```python
from build123d import *

# Parameters (mm, degrees)
SKETCH1_W           = 76.2
SKETCH1_H           = 25.4
SKETCH1_W_2         = 69.85
SKETCH1_H_2         = 19.05
EXTRUDE_THIN1_DEPTH = 38.1
SKETCH2_R           = 3.175
CUT_EXTRUDE1_DEPTH  = 77.2
SKETCH3_R           = 24.97201
CUT_EXTRUDE2_DEPTH  = 26.4


with BuildPart() as part:
    # Sketch1 → Extrude-Thin1 (new body, symmetric)
    with BuildSketch(Plane.XY):
        Rectangle(SKETCH1_W, SKETCH1_H)
        Rectangle(SKETCH1_W_2, SKETCH1_H_2, mode=Mode.SUBTRACT)
    extrude(amount=EXTRUDE_THIN1_DEPTH, both=True)

    # Sketch2 → Cut-Extrude1 (cut, through all)
    with BuildSketch(Plane.ZY.offset(38.1)):
        Circle(SKETCH2_R)
    extrude(amount=-CUT_EXTRUDE1_DEPTH, mode=Mode.SUBTRACT)

    # Sketch3 → Cut-Extrude2 (cut, through all)
    with BuildSketch(Plane(origin=(0, 12.7, 0), x_dir=(1, 0, 0), z_dir=(0, 1, 0))):
        Circle(SKETCH3_R)
    extrude(amount=-CUT_EXTRUDE2_DEPTH, mode=Mode.SUBTRACT)


solid = part.part
```
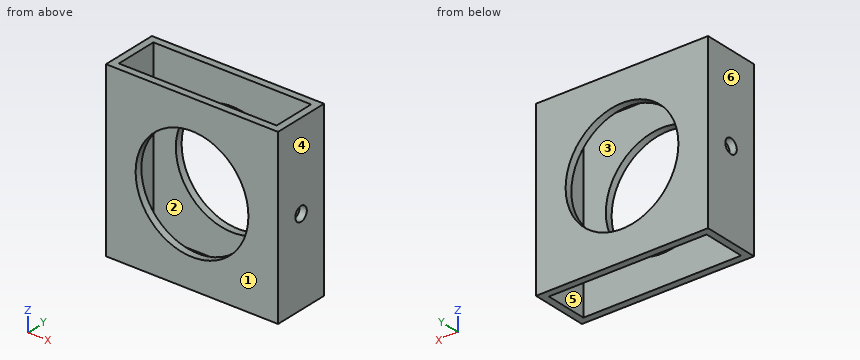
Design review of the part built by this model. Coordinates are the model's own, in mm. Face numbers are marked on the shaded views. A direction names the side the tool comes from. Coordinates: 2 decimals unless noted, no trailing zeros. Order: outer loops, then holes, each group sorted by start corner. A loop starts at its lowest first (then second) coordinate and runs counter-clockwise, first axis right, second up. Notation, with made-up numbers: (-8, 50.25) -> (32, 50.25) arc R27 cw to (32, 85.25) -> close; hole circle Ø1 at (0, 13). An arc over 180 degrees is marked (long way). One line per item, written item: value. Start each with the question number.
Q1. For probe 1 along X at (y, z) = (8, 32.5) (3 decimals); probe 2 along X at (y, z) = (-10.95, 0); probe 3 along Y at (x, z) = (23, -15) (3 decimals), list the stretches that pass through material, from the lowest coordinate up.
Q2. Tool access review of the marked faces 5 and 6: name each direction out of +Z, -Z, +X, -X, +Y, -Y from which nothing blocks a thin tool from reaching the whole face with its end or side.
Q3. Take a section at C-C, the plane z = 0. State the section outline as (x, y) points (3 decimals).
Q4. Take a section at B-B, the plane y = 0. State the section outline as (x, z) points (3 decimals).
Q5. Take a section at A-A, the plane x = 26. State the section outline as (y, z) points (3 decimals), then the cut area to 3 significant figures.
Q6. Take a section at D-D, the plane y = -6.5. State the section outline as (x, z) points (3 decimals), then the cut area to 3 significant figures.
Q7. Mouldability with a two-part tool opening along X and no side actions: class the marked faces 1, 2, 3 and 4 as pulls with the +X half, pulls with the -X half, needs draft (parallel to the pull), parting line crosses it, or undercut.
Values follow:
1. probe 1: x = -38.1 to -34.925, 34.925 to 38.1
1. probe 2: x = -38.1 to -24.97, 24.97 to 38.1
1. probe 3: y = -12.7 to -9.525, 9.525 to 12.7
2. face 5: +Z, -Z
2. face 6: +Z, -Z, -X, +Y, -Y
3. outline: (-38.1, -12.7) -> (-24.972, -12.7) -> (-24.972, -9.525) -> (-34.925, -9.525) -> (-34.925, -3.175) -> (-38.1, -3.175) -> close; (-38.1, 3.175) -> (-34.925, 3.175) -> (-34.925, 9.525) -> (-24.972, 9.525) -> (-24.972, 12.7) -> (-38.1, 12.7) -> close; (24.972, -12.7) -> (38.1, -12.7) -> (38.1, -3.175) -> (34.925, -3.175) -> (34.925, -9.525) -> (24.972, -9.525) -> close; (24.972, 9.525) -> (34.925, 9.525) -> (34.925, 3.175) -> (38.1, 3.175) -> (38.1, 12.7) -> (24.972, 12.7) -> close
4. outline: (-38.1, -38.1) -> (-34.925, -38.1) -> (-34.925, -3.175) -> (-38.1, -3.175) -> close; (-38.1, 3.175) -> (-34.925, 3.175) -> (-34.925, 38.1) -> (-38.1, 38.1) -> close; (34.925, -38.1) -> (38.1, -38.1) -> (38.1, -3.175) -> (34.925, -3.175) -> close; (34.925, 3.175) -> (38.1, 3.175) -> (38.1, 38.1) -> (34.925, 38.1) -> close
5. outline: (-12.7, -38.1) -> (-9.525, -38.1) -> (-9.525, 38.1) -> (-12.7, 38.1) -> close; (9.525, -38.1) -> (12.7, -38.1) -> (12.7, 38.1) -> (9.525, 38.1) -> close
5. area: 484 mm2
6. outline: (-38.1, -38.1) -> (-34.925, -38.1) -> (-34.925, 38.1) -> (-38.1, 38.1) -> close; (34.925, -38.1) -> (38.1, -38.1) -> (38.1, 38.1) -> (34.925, 38.1) -> close
6. area: 484 mm2
7. face 1: needs draft
7. face 2: undercut
7. face 3: undercut
7. face 4: pulls with the +X half
